Study the drawing (mm; zero at the part's minimum x, y, z) and answer. Give positions to 0.01 mm unless a question says otherwise; leave off trailing zeros. Order: outer loops, then holes, each group sorted by start corner. A loop starts at its lowest first (then second) coordinate and runs counter-clockwise, first axis right, second up.
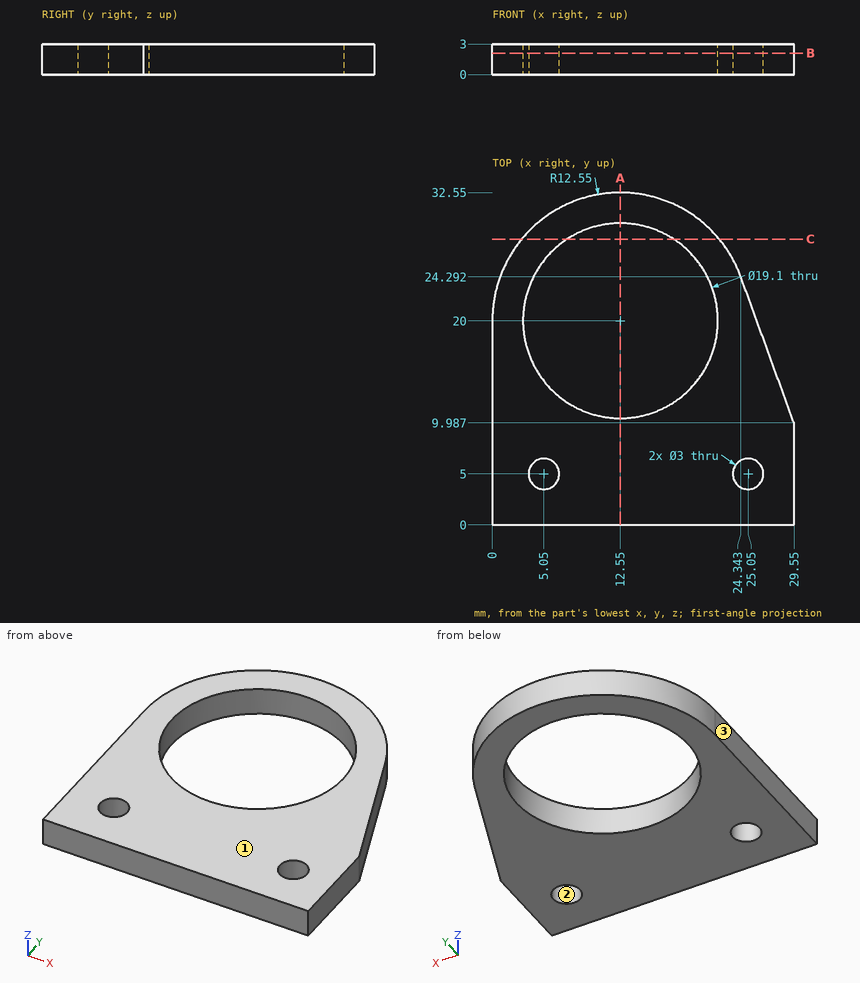
1) Find section B-B (z = 2.1). Write down the section's boundary in (x, y).
Geometry says:
outline: (0, 0) - (29.55, 0) - (29.55, 9.99) - (24.34, 24.29) arc R12.55 ccw to (0, 20) - close; hole circle Ø19.1 at (12.55, 20); hole circle Ø3 at (5.05, 5); hole circle Ø3 at (25.05, 5)
2) Straight lines are drawn through the part: probe 1 along Y at (x, z) = (5.05, 1.1) (1 decimal); probe 2 along Y at (x, z) = (18.5, 2.65); probe 3 along X at (y, z) = (10, 2.1) (1 decimal). For each, find the intervals that lie inside material, in ascending order.
Geometry says:
probe 1: y = 0 to 3.5, 6.5 to 14.1, 25.9 to 30.1
probe 2: y = 0 to 12.53, 27.47 to 31.05
probe 3: x = 0 to 29.5
3) Find section C-C (y = 28). Write down the section's boundary in (x, z) (1 decimal).
Geometry says:
outline: (2.9, 0) - (7.3, 0) - (7.3, 3) - (2.9, 3) - close; (17.8, 0) - (22.2, 0) - (22.2, 3) - (17.8, 3) - close
4) For a pull along X with two mould halves and no side action, classify the marked faces 1, 2 and 3 as +X half, -X half, draft (parallel to the pull), parting line (faces both ways), or undercut.
Geometry says:
face 1: draft
face 2: undercut
face 3: -X half
5) Given P1, Ø11.5, axis at x = 12.55, y = 20, coming from the -Z side; P2, Ø8, axis at x = 7.5, y = 12, coming from the +Z side, each flat-ended and moving along its own axis, determine where each tip first touches the part or whether it passes through.
Geometry says:
P1: passes through
P2: stops at z = 3
6) Find section A-A (x = 12.55). Write down the section's boundary in (y, z).
Geometry says:
outline: (0, 0) - (10.45, 0) - (10.45, 3) - (0, 3) - close; (29.55, 0) - (32.55, 0) - (32.55, 3) - (29.55, 3) - close
